from build123d import *

# Parameters (mm, degrees)
BOSS_EXTRUDE1_DEPTH = 6.223


with BuildPart() as part:
    # Sketch1 → Boss-Extrude1 (new body)
    with BuildSketch(Plane.XY):
        with BuildLine():
            ThreePointArc((32.995567884, 38.1), (-34.813454061, 34.530097426), (7.956908754, -18.209865849))
            Line((7.956908754, -18.209865849), (-14.14476943, 6.28959257))
            Line((-14.14476943, 6.28959257), (-2.310313541, 16.965801451))
            ThreePointArc((-2.310313541, 16.965801451), (-2.843098313, 20.314208935), (0, 22.1615))
            Line((0, 22.1615), (0, 38.1))
            Line((0, 38.1), (32.995567884, 38.1))
        make_face()
        with BuildLine():
            Line((14.14476656, 31.810410611), (36.246444744, 7.310952192))
            ThreePointArc((36.246444744, 7.310952192), (37.633758414, 13.10775904), (38.1, 19.05))
            ThreePointArc((38.1, 19.05), (36.801773982, 28.911005618), (32.995567884, 38.1))
            Line((32.995567884, 38.1), (0, 38.1))
            Line((0, 38.1), (0, 22.1615))
            ThreePointArc((0, 22.1615), (1.264206978, 21.893099184), (2.310310671, 21.134201731))
            Line((2.310310671, 21.134201731), (14.14476656, 31.810410611))
        make_face()
        with BuildLine():
            Line((0, 15.9385), (0, 0))
            Line((0, 0), (32.995567884, 0))
            ThreePointArc((32.995567884, 0), (34.813454061, 3.569902574), (36.246444744, 7.310952192))
            Line((36.246444744, 7.310952192), (14.14476656, 31.810410611))
            Line((14.14476656, 31.810410611), (2.310310671, 21.134201731))
            ThreePointArc((2.310310671, 21.134201731), (2.904304039, 20.166445385), (3.1115, 19.05))
            ThreePointArc((3.1115, 19.05), (2.20016275, 16.84983725), (0, 15.9385))
        make_face()
        with BuildLine():
            Line((32.995567884, 0), (0, 0))
            Line((0, 0), (0, 15.9385))
            ThreePointArc((0, 15.9385), (-1.264208935, 16.206901687), (-2.310313541, 16.965801451))
            Line((-2.310313541, 16.965801451), (-14.14476943, 6.28959257))
            Line((-14.14476943, 6.28959257), (7.956908754, -18.209865849))
            ThreePointArc((7.956908754, -18.209865849), (22.409286898, -11.762884655), (32.995567884, 0))
        make_face()
        with BuildLine():
            Line((36.246444744, 7.310952192), (42.841868602, 0))
            Line((42.841868602, 0), (191.108363525, 0))
            Line((191.108363525, 0), (199.557192075, 8.684262446))
            ThreePointArc((199.557192075, 8.684262446), (198.412676185, 23.763413406), (203.224432116, 38.1))
            Line((203.224432116, 38.1), (32.995567884, 38.1))
            ThreePointArc((32.995567884, 38.1), (36.801773982, 28.911005618), (38.1, 19.05))
            ThreePointArc((38.1, 19.05), (37.633758414, 13.10775904), (36.246444744, 7.310952192))
        make_face()
        with BuildLine():
            ThreePointArc((36.246444744, 7.310952192), (34.813454061, 3.569902574), (32.995567884, 0))
            Line((32.995567884, 0), (42.841868602, 0))
            Line((42.841868602, 0), (36.246444744, 7.310952192))
        make_face()
        with BuildLine():
            Line((42.841868602, 0), (32.995567884, 0))
            ThreePointArc((32.995567884, 0), (22.409286898, -11.762884655), (7.956908754, -18.209865849))
            Line((7.956908754, -18.209865849), (77.406264934, -95.193685799))
            ThreePointArc((77.406264934, -95.193685799), (88.131891636, -78.643197617), (105.695800923, -69.672867758))
            Line((105.695800923, -69.672867758), (42.841868602, 0))
        make_face()
        with BuildLine():
            ThreePointArc((203.224432116, 38.1), (198.412676185, 23.763413406), (199.557192075, 8.684262446))
            Line((199.557192075, 8.684262446), (222.565801994, 32.33402713))
            Line((222.565801994, 32.33402713), (233.989814326, 21.219724431))
            ThreePointArc((233.989814326, 21.219724431), (235.00955903, 21.916402782), (236.22, 22.1615))
            Line((236.22, 22.1615), (236.22, 38.1))
            Line((236.22, 38.1), (203.224432116, 38.1))
        make_face()
        with BuildLine():
            Line((199.557192075, 8.684262446), (191.108363525, 0))
            Line((191.108363525, 0), (203.224432116, 0))
            ThreePointArc((203.224432116, 0), (201.121190424, 4.228273841), (199.557192075, 8.684262446))
        make_face()
        with BuildLine():
            ThreePointArc((199.557192075, 8.684262446), (201.121190424, 4.228273841), (203.224432116, 0))
            Line((203.224432116, 0), (236.22, 0))
            Line((236.22, 0), (236.22, 15.9385))
            ThreePointArc((236.22, 15.9385), (233.353597218, 17.83955903), (233.989814326, 21.219724431))
            Line((233.989814326, 21.219724431), (222.565801994, 32.33402713))
            Line((222.565801994, 32.33402713), (199.557192075, 8.684262446))
        make_face()
        with BuildLine():
            ThreePointArc((274.32, 19.05), (246.081005618, 55.851773982), (203.224432116, 38.1))
            Line((203.224432116, 38.1), (236.22, 38.1))
            Line((236.22, 38.1), (236.22, 22.1615))
            ThreePointArc((236.22, 22.1615), (238.42016275, 21.25016275), (239.3315, 19.05))
            ThreePointArc((239.3315, 19.05), (239.102763863, 17.879058173), (238.450185674, 16.880275569))
            Line((238.450185674, 16.880275569), (249.874198006, 5.76597287))
            Line((249.874198006, 5.76597287), (226.865588088, -17.883791814))
            ThreePointArc((226.865588088, -17.883791814), (259.620928466, -11.01670163), (274.32, 19.05))
        make_face()
        with BuildLine():
            Line((236.22, 0), (203.224432116, 0))
            ThreePointArc((203.224432116, 0), (213.234402344, -11.33539617), (226.865588088, -17.883791814))
            Line((226.865588088, -17.883791814), (249.874198006, 5.76597287))
            Line((249.874198006, 5.76597287), (238.450185674, 16.880275569))
            ThreePointArc((238.450185674, 16.880275569), (237.43044097, 16.183597218), (236.22, 15.9385))
            Line((236.22, 15.9385), (236.22, 0))
        make_face()
        with BuildLine():
            Line((203.224432116, 0), (191.108363525, 0))
            Line((191.108363525, 0), (123.00712159, -69.998941792))
            ThreePointArc((123.00712159, -69.998941792), (140.220763938, -79.624337594), (150.315517603, -96.566996053))
            Line((150.315517603, -96.566996053), (226.865588088, -17.883791814))
            ThreePointArc((226.865588088, -17.883791814), (213.234402344, -11.33539617), (203.224432116, 0))
        make_face()
        with BuildLine():
            ThreePointArc((123.00712159, -69.998941792), (114.370229599, -68.839490568), (105.695800923, -69.672867758))
            Line((105.695800923, -69.672867758), (114.17744096, -79.07466909))
            Line((114.17744096, -79.07466909), (123.00712159, -69.998941792))
        make_face()
        with BuildLine():
            Line((114.17744096, -79.07466909), (105.695800923, -69.672867758))
            ThreePointArc((105.695800923, -69.672867758), (88.131891636, -78.643197617), (77.406264934, -95.193685799))
            Line((77.406264934, -95.193685799), (99.507943118, -119.693144218))
            Line((99.507943118, -119.693144218), (111.342399007, -109.016935337))
            ThreePointArc((111.342399007, -109.016935337), (110.541761476, -106.874137217), (111.422524003, -104.763009175))
            Line((111.422524003, -104.763009175), (99.998511671, -93.648706476))
            Line((99.998511671, -93.648706476), (114.17744096, -79.07466909))
        make_face()
        with BuildLine():
            Line((127.797479107, -94.172326176), (114.17744096, -79.07466909))
            Line((114.17744096, -79.07466909), (99.998511671, -93.648706476))
            Line((99.998511671, -93.648706476), (111.422524003, -104.763009175))
            ThreePointArc((111.422524003, -104.763009175), (113.711308209, -103.821785445), (115.963023218, -104.848535057))
            Line((115.963023218, -104.848535057), (127.797479107, -94.172326176))
        make_face()
        with BuildLine():
            ThreePointArc((150.315517603, -96.566996053), (140.220763938, -79.624337594), (123.00712159, -69.998941792))
            Line((123.00712159, -69.998941792), (114.17744096, -79.07466909))
            Line((114.17744096, -79.07466909), (127.797479107, -94.172326176))
            Line((127.797479107, -94.172326176), (115.963023218, -104.848535057))
            ThreePointArc((115.963023218, -104.848535057), (116.557014485, -105.816290221), (116.764209677, -106.932733607))
            ThreePointArc((116.764209677, -106.932733607), (116.53547354, -108.103675433), (115.882895352, -109.102458038))
            Line((115.882895352, -109.102458038), (127.306907684, -120.216760737))
            Line((127.306907684, -120.216760737), (150.315517603, -96.566996053))
        make_face()
        with BuildLine():
            Line((99.507943118, -119.693144218), (77.406264934, -95.193685799))
            ThreePointArc((77.406264934, -95.193685799), (107.710468717, -144.566492021), (151.752709677, -106.932733607))
            ThreePointArc((151.752709677, -106.932733607), (151.39170133, -101.700285898), (150.315517603, -96.566996053))
            Line((150.315517603, -96.566996053), (127.306907684, -120.216760737))
            Line((127.306907684, -120.216760737), (115.882895352, -109.102458038))
            ThreePointArc((115.882895352, -109.102458038), (113.594113288, -110.043681808), (111.342399007, -109.016935337))
            Line((111.342399007, -109.016935337), (99.507943118, -119.693144218))
        make_face()
    extrude(amount=-BOSS_EXTRUDE1_DEPTH)


solid = part.part
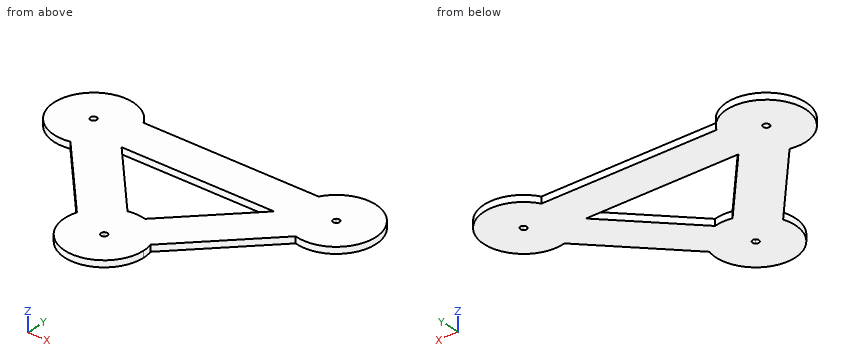
Source: CAD feature listing. Evaluate the final solid. Frame: model axes, mm. Coordinates: 2 decimals unless noted, no trailing zeros. Loops run counter-clockwise (first coordinate to the right, second up) from the corner with the lowest first, then second, coordinate; pieces in that order, holes last. Notation, with made-up numbers: (55.5, 87.5) - (82.5, 87.5) arc R16 cw to (82.5, 107.5) - close; hole circle Ø9 at (69, 78). An arc over 180 degrees is marked (long way). One line per question, with ' | ' between items.
1) Line query: line 1 along X through (y, z) = (21, -1); line 2 along Y through (x, z) = (144, -1.25); line 3 along X through (y, z) = (-34.5, -3.5). Output: solid intervals per line, ascending.
Report:
line 1: x = -38.05 to -2.42, 2.42 to 233.8, 238.64 to 274.27 | line 2: y = -129.97 to -48.42, 0 to 38.1 | line 3: x = 22.65 to 73.97, 157.54 to 210.7
2) Section B-B, the plane x = 139. Return loops of the section in (y, z), then the cut area to 3 significant figures.
Report:
outline: (-135.38, -6.22) - (-53.56, -6.22) - (-53.56, 0) - (-135.38, 0) - close; (0, -6.22) - (38.1, -6.22) - (38.1, 0) - (0, 0) - close | area: 746 mm²
3) Section A-A, the plane z = -2. Return loops of the section in (x, y), then the cut area to 3 significant figures.
Report:
outline: (7.96, -18.21) - (77.41, -95.19) arc R38.1 ccw (long way) to (150.32, -96.57) - (226.87, -17.88) arc R38.1 ccw (long way) to (203.22, 38.1) - (33, 38.1) arc R38.1 ccw (long way) to start; hole circle Ø6.22 at (0, 19.05); hole (42.84, 0) - (105.7, -69.67) arc R38.1 cw to (123.01, -70) - (191.11, 0) - close; hole circle Ø6.22 at (113.65, -106.93); hole circle Ø6.22 at (236.22, 19.05) | area: 27,300 mm²
4) Section D-D, the plane y = -125.5. Return loops of the section in (x, z), then the cut area to 3 significant figures.
Report:
outline: (80.38, -6.22) - (146.92, -6.22) - (146.92, 0) - (80.38, 0) - close | area: 414 mm²
5) First-contact query: P1, Ø2, axis at x = 164, z = -4.5, coming from the +Y side; P2, Ø1.5, axis at x = 214.5, z = -3, coming from the -Y side. Flat tips, straight axial feed; report the tip coordinate or a pass-through.
Report:
P1: stops at y = 38.1 | P2: stops at y = -31.36
6) Section C-C, the plane y = -46. Return loops of the section in (x, z), then the cut area to 3 significant figures.
Report:
outline: (33.03, -6.22) - (84.34, -6.22) - (84.34, 0) - (33.03, 0) - close; (146.36, -6.22) - (199.51, -6.22) - (199.51, 0) - (146.36, 0) - close | area: 650 mm²
